from build123d import *

# Parameters (mm, degrees)
BOSS_EXTRUDE1_DEPTH      = 10
CUT_EXTRUDE3_DEPTH       = 5
BOSS_EXTRUDE6_DEPTH      = 5
BOSS_EXTRUDE6_DEPTH_BACK = 10
SKETCH5_W                = 4.5
SKETCH5_H                = 5
CUT_EXTRUDE5_DEPTH       = 60
CUT_EXTRUDE7_DEPTH       = 5


with BuildPart() as part:
    # Sketch1 → Boss-Extrude1 (new body)
    with BuildSketch(Plane(origin=(0, 0, 0), x_dir=(1, 0, 0), z_dir=(0, 1, 0))):
        with BuildLine():
            Line((-23.3656, -38.85), (16.6344, -38.85))
            ThreePointArc((16.6344, -38.85), (19.816380515, -37.531980515), (21.1344, -34.35))
            Line((21.1344, -34.35), (21.1344, 34.35))
            ThreePointArc((21.1344, 34.35), (19.816380515, 37.531980515), (16.6344, 38.85))
            Line((16.6344, 38.85), (-23.3656, 38.85))
            ThreePointArc((-23.3656, 38.85), (-26.547580515, 37.531980515), (-27.8656, 34.35))
            Line((-27.8656, 34.35), (-27.8656, -34.35))
            ThreePointArc((-27.8656, -34.35), (-26.547580515, -37.531980515), (-23.3656, -38.85))
        make_face()
    extrude(amount=BOSS_EXTRUDE1_DEPTH)

    # Sketch2 → Cut-Extrude3 (cut)
    with BuildSketch(Plane(origin=(0, 10, 0), x_dir=(1, 0, 0), z_dir=(0, 1, 0))):
        with BuildLine():
            Line((-23.0156, -14.55), (-27.8656, -14.55))
            Line((-27.8656, -14.55), (-27.8656, -28.75))
            ThreePointArc((-27.8656, -28.75), (-26.547580515, -25.568019485), (-23.3656, -24.25))
            Line((-23.3656, -24.25), (16.6344, -24.25))
            ThreePointArc((16.6344, -24.25), (19.816380515, -25.568019485), (21.1344, -28.75))
            Line((21.1344, -28.75), (21.1344, -14.55))
            Line((21.1344, -14.55), (16.2844, -14.55))
            Line((16.2844, -14.55), (-23.0156, -14.55))
        make_face()
        with BuildLine():
            ThreePointArc((-23.0156, -14.55), (-26.445067903, -13.129467874), (-27.8656, -9.699999958))
            Line((-27.8656, -9.699999958), (-27.8656, -14.55))
            Line((-27.8656, -14.55), (-23.0156, -14.55))
        make_face()
        with BuildLine():
            Line((21.1344, -14.55), (21.1344, -9.7))
            ThreePointArc((21.1344, -9.7), (19.713867889, -13.129467889), (16.2844, -14.55))
            Line((16.2844, -14.55), (21.1344, -14.55))
        make_face()
        with BuildLine():
            Line((21.1344, -9.7), (21.1344, -4.85))
            Line((21.1344, -4.85), (16.28440001, -4.85))
            ThreePointArc((16.28440001, -4.85), (19.713867892, -6.270532115), (21.1344, -9.7))
        make_face()
        with BuildLine():
            Line((-23.0156, -4.85), (-27.8656, -4.85))
            Line((-27.8656, -4.85), (-27.8656, -9.699999958))
            ThreePointArc((-27.8656, -9.699999958), (-26.445067874, -6.270532097), (-23.0156, -4.85))
        make_face()
        Polygon((-23.0156, 4.85), (-27.8656, 4.85), (-27.8656, -4.85), (-23.0156, -4.85), (16.28440001, -4.85), (21.1344, -4.85), (21.1344, 4.85), (16.284399974, 4.85), align=None)
        with BuildLine():
            ThreePointArc((-23.0156, 4.85), (-26.445067902, 6.270532124), (-27.8656, 9.700000036))
            Line((-27.8656, 9.700000036), (-27.8656, 4.85))
            Line((-27.8656, 4.85), (-23.0156, 4.85))
        make_face()
        with BuildLine():
            Line((21.1344, 4.85), (21.1344, 9.7))
            ThreePointArc((21.1344, 9.7), (19.71386788, 6.270532102), (16.284399974, 4.85))
            Line((16.284399974, 4.85), (21.1344, 4.85))
        make_face()
        with BuildLine():
            Line((-23.015600011, 14.55), (-27.8656, 14.55))
            Line((-27.8656, 14.55), (-27.8656, 9.700000036))
            ThreePointArc((-27.8656, 9.700000036), (-26.44506788, 13.129467898), (-23.015600011, 14.55))
        make_face()
        with BuildLine():
            Line((16.6344, 24.25), (-23.3656, 24.25))
            ThreePointArc((-23.3656, 24.25), (-26.547580515, 25.568019485), (-27.8656, 28.75))
            Line((-27.8656, 28.75), (-27.8656, 14.55))
            Line((-27.8656, 14.55), (-23.015600011, 14.55))
            Line((-23.015600011, 14.55), (16.2844, 14.55))
            Line((16.2844, 14.55), (21.1344, 14.55))
            Line((21.1344, 14.55), (21.1344, 28.75))
            ThreePointArc((21.1344, 28.75), (19.816380515, 25.568019485), (16.6344, 24.25))
        make_face()
        with BuildLine():
            Line((21.1344, 9.7), (21.1344, 14.55))
            Line((21.1344, 14.55), (16.2844, 14.55))
            ThreePointArc((16.2844, 14.55), (19.713867889, 13.129467889), (21.1344, 9.7))
        make_face()
    extrude(amount=-CUT_EXTRUDE3_DEPTH, mode=Mode.SUBTRACT)

    # Sketch4 → Boss-Extrude6 (add, two sides: drawn at the far end of the back side and taken through both)
    with BuildSketch(Plane.XZ.offset(-BOSS_EXTRUDE6_DEPTH_BACK)):
        with BuildLine():
            ThreePointArc((-27.8656, 34.35), (-26.547580515, 37.531980515), (-23.3656, 38.85))
            Line((-23.3656, 38.85), (-27.8656, 38.85))
            Line((-27.8656, 38.85), (-27.8656, 34.35))
        make_face()
        with BuildLine():
            Line((-23.3656, 35.615611346), (-23.3656, 38.85))
            ThreePointArc((-23.3656, 38.85), (-26.547580515, 37.531980515), (-27.8656, 34.35))
            Line((-27.8656, 34.35), (-27.8656, 34.176611106))
            Line((-27.8656, 34.176611106), (-23.3656, 35.615611346))
        make_face()
        with BuildLine():
            Line((17.428758808, 36.847416441), (16.6344, 38.85))
            ThreePointArc((16.6344, 38.85), (19.816380515, 37.531980515), (21.1344, 34.35))
            Line((21.1344, 34.35), (17.428758808, 36.847416441))
        make_face()
        with BuildLine():
            Line((21.1344, 38.85), (21.1344, 34.35))
            ThreePointArc((21.1344, 34.35), (19.816380515, 37.531980515), (16.6344, 38.85))
            Line((16.6344, 38.85), (21.1344, 38.85))
        make_face()
        with BuildLine():
            Line((16.6344, -34.745010915), (21.1344, -34.35))
            ThreePointArc((21.1344, -34.35), (19.816380515, -37.531980515), (16.6344, -38.85))
            Line((16.6344, -38.85), (16.6344, -34.745010915))
        make_face()
        with BuildLine():
            Line((16.6344, -38.85), (21.1344, -38.85))
            Line((21.1344, -38.85), (21.1344, -34.35))
            ThreePointArc((21.1344, -34.35), (19.816380515, -37.531980515), (16.6344, -38.85))
        make_face()
        with BuildLine():
            Line((-23.3656, -38.85), (-23.156696732, -35.585785164))
            Line((-23.156696732, -35.585785164), (-27.8656, -34.35))
            ThreePointArc((-27.8656, -34.35), (-26.547580515, -37.531980515), (-23.3656, -38.85))
        make_face()
        with BuildLine():
            Line((-27.8656, -34.35), (-27.8656, -38.85))
            Line((-27.8656, -38.85), (-23.3656, -38.85))
            ThreePointArc((-23.3656, -38.85), (-26.547580515, -37.531980515), (-27.8656, -34.35))
        make_face()
    extrude(amount=BOSS_EXTRUDE6_DEPTH + BOSS_EXTRUDE6_DEPTH_BACK)

    # Sketch5 → Cut-Extrude5 (cut)
    with BuildSketch(Plane(origin=(21.1344, 0, 0), x_dir=(0, 0, -1), z_dir=(1, 0, 0))):
        Polygon((34.35, 0), (-34.35, 0), (-34.35, -5), (-38.85, -5), (-38.85, -11.467862175), (41.584838498, -11.467862175), (41.584838498, 0), (38.85, 0), (38.85, -5), (34.35, -5), align=None)
        with Locations((36.6, -2.5)):
            Rectangle(SKETCH5_W, SKETCH5_H)
        with Locations((-36.6, -2.5)):
            Rectangle(SKETCH5_W, SKETCH5_H)
    extrude(amount=-CUT_EXTRUDE5_DEPTH, mode=Mode.SUBTRACT)

    # Sketch6 → Cut-Extrude7 (cut)
    with BuildSketch(Plane.XZ):
        with BuildLine():
            ThreePointArc((-27.8656, 34.05), (-26.45971255, 37.44411255), (-23.0656, 38.85))
            Line((-23.0656, 38.85), (-27.8656, 38.85))
            Line((-27.8656, 38.85), (-27.8656, 34.05))
        make_face()
        with BuildLine():
            Line((-18.2656, 34.05), (-18.2656, 38.85))
            Line((-18.2656, 38.85), (-23.0656, 38.85))
            ThreePointArc((-23.0656, 38.85), (-19.67148745, 37.44411255), (-18.2656, 34.05))
        make_face()
        Polygon((-8.2656, 38.85), (-18.2656, 38.85), (-18.2656, 34.05), (-18.2656, -34.05), (-18.2656, -38.85), (-8.2656, -38.85), (-8.2656, -33.950000026), (-8.2656, 33.95), align=None)
        with BuildLine():
            Line((-3.365599985, 38.85), (-8.2656, 38.85))
            Line((-8.2656, 38.85), (-8.2656, 33.95))
            ThreePointArc((-8.2656, 33.95), (-6.830423222, 37.414823233), (-3.365599985, 38.85))
        make_face()
        with BuildLine():
            Line((1.5344, 38.85), (-3.365599985, 38.85))
            ThreePointArc((-3.365599985, 38.85), (0.099223233, 37.414823222), (1.5344, 33.95))
            Line((1.5344, 33.95), (1.5344, 38.85))
        make_face()
        Polygon((1.5344, 38.85), (1.5344, 33.95), (1.5344, -33.95), (1.5344, -38.85), (11.5344, -38.85), (11.5344, -34.050000018), (11.5344, 34.05), (11.5344, 38.85), align=None)
        with BuildLine():
            Line((16.3344, 38.85), (11.5344, 38.85))
            Line((11.5344, 38.85), (11.5344, 34.05))
            ThreePointArc((11.5344, 34.05), (12.94028745, 37.44411255), (16.3344, 38.85))
        make_face()
        with BuildLine():
            Line((21.1344, 38.85), (16.3344, 38.85))
            ThreePointArc((16.3344, 38.85), (19.72851255, 37.44411255), (21.1344, 34.05))
            Line((21.1344, 34.05), (21.1344, 38.85))
        make_face()
        with BuildLine():
            ThreePointArc((21.1344, -34.05), (19.72851255, -37.44411255), (16.3344, -38.85))
            Line((16.3344, -38.85), (21.1344, -38.85))
            Line((21.1344, -38.85), (21.1344, -34.05))
        make_face()
        with BuildLine():
            Line((11.5344, -34.050000018), (11.5344, -38.85))
            Line((11.5344, -38.85), (16.3344, -38.85))
            ThreePointArc((16.3344, -38.85), (12.940287457, -37.444112556), (11.5344, -34.050000018))
        make_face()
        with BuildLine():
            Line((1.5344, -38.85), (1.5344, -33.95))
            ThreePointArc((1.5344, -33.95), (0.099223245, -37.414823211), (-3.365599951, -38.85))
            Line((-3.365599951, -38.85), (1.5344, -38.85))
        make_face()
        with BuildLine():
            ThreePointArc((-3.365599951, -38.85), (-6.830423201, -37.414823254), (-8.2656, -33.950000026))
            Line((-8.2656, -33.950000026), (-8.2656, -38.85))
            Line((-8.2656, -38.85), (-3.365599951, -38.85))
        make_face()
        with BuildLine():
            Line((-18.2656, -38.85), (-18.2656, -34.05))
            ThreePointArc((-18.2656, -34.05), (-19.67148745, -37.44411255), (-23.0656, -38.85))
            Line((-23.0656, -38.85), (-18.2656, -38.85))
        make_face()
        with BuildLine():
            ThreePointArc((-23.0656, -38.85), (-26.459712556, -37.444112543), (-27.8656, -34.049999982))
            Line((-27.8656, -34.049999982), (-27.8656, -38.85))
            Line((-27.8656, -38.85), (-23.0656, -38.85))
        make_face()
    extrude(amount=-CUT_EXTRUDE7_DEPTH, mode=Mode.SUBTRACT)


solid = part.part
Model file for the job. Use its own axes, mm. A direction names the side the tool comes from. Round coordinates to 2 decimals unless told otherwise and drop trailing zeros. Loops run counter-clockwise (first coordinate to the right, second up) from the corner with the lowest first, then second, coordinate; pieces in that order, holes last. Notation, with made-up numbers: M 68,-15 L 73,-15 A21 cw 73,21 Z; hole C -2,35.25 d11. An arc over 180 degrees is marked long. One line per question, with ' | ' between items.
1) Band-saw the part on C-C (z = 22.5). Give the cut face in (x, y), then the cut area to 3 significant figures.
Solved:
outline: M -27.87,0 L -18.27,0 L -18.27,5 L -27.87,5 Z; M -8.27,0 L 1.53,0 L 1.53,5 L -8.27,5 Z; M 11.53,0 L 21.13,0 L 21.13,5 L 11.53,5 Z | area: 145 mm²
2) Mould opens along Z. For faces 1 (the flat face through (-8.266, 2, 0)), 2 (the flat face through (-3, 7, -38.85)), 3 (the flat face through (-3, 8, -24.25)), 4 (the flat face through (-3, 5, -19)) say: +Z half, -Z half, draft (parallel to the pull), parting line (faces both ways), or undercut.
Solved:
face 1: draft | face 2: -Z half | face 3: undercut | face 4: undercut
3) Band-saw the part on D-D (y = 3). Give the cut face in (x, z), then the cut area to 3 significant figures.
Solved:
outline: M -27.87,-34.05 A4.8 ccw -18.27,-34.05 L -18.27,34.05 A4.8 ccw -27.87,34.05 Z; M -8.27,-33.95 A4.9 ccw 1.53,-33.95 L 1.53,33.95 A4.9 ccw -8.27,33.95 Z; M 11.53,-34.05 A4.8 ccw 21.13,-34.05 L 21.13,34.05 A4.8 ccw 11.53,34.05 Z | area: 2,190 mm²
4) Band-saw the part on B-B (x = -15.5). Give the cut face in (y, z), then the cut area to 3 significant figures.
Solved:
outline: M 5,-38.85 L 10,-38.85 L 10,-24.25 L 5,-24.25 Z; M 5,-14.55 L 10,-14.55 L 10,-4.85 L 5,-4.85 Z; M 5,4.85 L 10,4.85 L 10,14.55 L 5,14.55 Z; M 5,24.25 L 10,24.25 L 10,38.85 L 5,38.85 Z | area: 243 mm²
5) Flat gauge pins, fed straight in: pin 1 (7.5 mm diameter, centred on x = 5, z = -31.5, fed in from -Y); pin 2 (1 mm diameter, centred on x = -10, z = 24.5, fed in from -Y); pin 3 (3 mm diameter, centred on x = -3.5, z = -20, fed in from +Y). Where does each tip first touch, or does it go through?
Solved:
pin 1: stops at y = 0 | pin 2: stops at y = 5 | pin 3: stops at y = 5
6) 3-axis set-ups, long thin cutter, end or side, ignore diameter. For faces 5 (the cylindrical face through (19.78, 7.54, 25.53)), 6 (the flat face through (-13, 5, 10)), 7 (the flat face through (-27, 5, -38)), 8 (the flat face through (20, 5, 38)): which of +Z, -Z, +X, -X, +Y, -Y reach the whole face in a straight line?
Solved:
face 5: +X, +Y | face 6: +Z, -Z, -Y | face 7: -Z, -X, -Y | face 8: +Z, +X, -Y
7) Drill centre lines: line 1 along X through (y, z) = (3.25, 15); line 2 along Z through (x, y) = (-13, 6). Where is each one in solid material? Low to high.
Solved:
line 1: x = -27.87 to -18.27, -8.27 to 1.53, 11.53 to 21.13 | line 2: z = -38.85 to -24.25, -14.55 to -4.85, 4.85 to 14.55, 24.25 to 38.85
8) Band-saw the part on A-A (y = 7.5). Give the cut face in (x, z).
Solved:
outline: M -27.87,-38.85 L 21.13,-38.85 L 21.13,-28.75 A4.5 ccw 16.63,-24.25 L -23.37,-24.25 A4.5 ccw -27.87,-28.75 Z; M -27.87,28.75 A4.5 ccw -23.37,24.25 L 16.63,24.25 A4.5 ccw 21.13,28.75 L 21.13,38.85 L -27.87,38.85 Z; M -23.02,-14.55 L 16.28,-14.55 A4.85 ccw 16.28,-4.85 L -23.02,-4.85 A4.85 ccw Z; M -23.02,4.85 L 16.28,4.85 A4.85 ccw 16.28,14.55 L -23.02,14.55 A4.85 ccw Z
